Geometry: final body of the model. Coordinates: model frame, mm. A direction names the side the tool comes from. Give positions to 0.01 mm unless a question says otherwise; leave off trailing zeros. Write each loop counter-clockwise with the first axis right and the second up, starting at its lowest first coordinate (ties: lowest second). Pieces come first, ordered by that corner, then holes. Notation, with made-up numbers: M 1.25,5 L 22.25,5 A8 cw 22.25,14 Z; hole C 52,19 d1. An arc over 180 degrees is marked long. Answer as a JSON object with one key per item and string values.
Autodesk Inventor part; units mm, degrees
ref_plane "YZ Plane" through (0, 0, 0) normal (1, 0, 0) x (0, 1, 0)
ref_plane "XZ Plane" through (0, 0, 0) normal (0, 1, 0) x (-1, 0, 0)
ref_plane "XY Plane" through (0, 0, 0) normal (0, 0, 1) x (1, 0, 0)
sketch "スケッチ1" plane through (0, 0, 0) normal (0, 1, 0) x (-1, 0, 0)
  line L0 (-88.25, 46.25) -> (88.25, 46.25)
  line L1 (88.25, 46.25) -> (88.25, -46.25)
  line L2 (88.25, -46.25) -> (-88.25, -46.25)
  line L3 (-88.25, -46.25) -> (-88.25, 46.25)
  line L4 (-88.25, 46.25) -> (88.25, -46.25) construction
  line L5 (88.25, 46.25) -> (-88.25, -46.25) construction
  circle A0 centre (84.75, 42.75) radius 1.55
  circle A1 centre (9.75, 42.75) radius 1.55
  circle A2 centre (-84.75, 42.75) radius 1.55
  line L6 (151.0272, 0) -> (-157.6431, 0) construction
  line L7 (0, 129.3763) -> (0, -94.6315) construction
  circle A3 centre (84.75, -42.75) radius 1.55
  circle A4 centre (9.75, -42.75) radius 1.55
  circle A5 centre (-84.75, -42.75) radius 1.55
  circle A6 centre (30, -25.75) radius 1.55
  circle A7 centre (30, -16.25) radius 1.55
  line L8 (88.25, -25.75) -> (-88.25, -25.75) construction
  line L9 (-88.25, -16.25) -> (88.25, -16.25) construction
  circle A8 centre (-69.5, -25.75) radius 1.55
  circle A9 centre (-69.5, -16.25) radius 1.55
  circle A10 centre (84.75, -29.75) radius 1.55
  circle A11 centre (84.75, -14.75) radius 1.55
  circle A12 centre (84.75, 0.25) radius 1.55
  circle A13 centre (84.75, 15.25) radius 1.55
  circle A14 centre (84.75, 30.25) radius 1.55
  circle A15 centre (76.5, -25.75) radius 1.55
  circle A16 centre (76.5, -13.75) radius 1.55
  circle A17 centre (76.5, -1.75) radius 1.55
  circle A18 centre (76.5, 10.25) radius 1.55
  line L10 (-55.5, -30.75) -> (24.5, -30.75)
  line L11 (24.5, -30.75) -> (24.5, 29.25)
  line L12 (24.5, 29.25) -> (-55.5, 29.25)
  line L13 (-55.5, 29.25) -> (-55.5, -30.75)
  line L14 (-55.5, -30.75) -> (24.5, 29.25) construction
  line L15 (24.5, -30.75) -> (-55.5, 29.25) construction
  point P0 (0, 0)
  point P1 (-15.5, -0.75)
  dimension "d105" = 176.5
  dimension "d106" = 92.5
  dimension "d107" = 3.5
  dimension "d108" = 3.5
  dimension "d109" = 3.1
  dimension "d110" = 78.5
  dimension "d111" = 3.5
  dimension "d112" = 3.1
  dimension "d113" = 173
  dimension "d114" = 3.5
  dimension "d115" = 3.1
  dimension "d116" = 46.25
  dimension "d117" = 88.25
  dimension "d118" = 58.25
  dimension "d119" = 20.5
  dimension "d120" = 30
  dimension "d121" = 3.1
  dimension "d122" = 3.1
  dimension "d123" = 58.25
  dimension "d129" = 3.1
  dimension "d130" = 3.1
  dimension "d132" = 9.5
  dimension "d133" = 20.5
  dimension "d134" = 30
  dimension "d136" = 16.5
  dimension "d137" = 3.5
  dimension "d138" = 3.1
  dimension "d141" = 15
  dimension "d146" = 20.5
  dimension "d147" = 11.75
  dimension "d148" = 3.1
  dimension "d151" = 12
  dimension "d156" = 15.5
  dimension "d157" = 75.5
  dimension "d158" = 63.75
  dimension "d159" = 143.75
  dimension "d164" = 99.5
  dimension "d165" = 157.75
extrude "押し出し1" add sketch "スケッチ1" along normal blind 3
fillet "フィレット1" radius 2 4 edges at (-24.5, 1.5, 29.25) (-24.5, 1.5, -30.75) (55.5, 1.5, 29.25) (55.5, 1.5, -30.75)
fillet "フィレット2" radius 3 4 edges at (-88.25, 1.5, 46.25) (-88.25, 1.5, -46.25) (88.25, 1.5, 46.25) (88.25, 1.5, -46.25)
equation "\"d108\" = d107"
equation "\"d111\" = d107"
equation "\"d112\" = d109"
equation "\"d114\" = d111"
equation "\"d115\" = d112"
equation "\"d121\" = d109"
equation "\"d122\" = d109"
equation "\"d123\" = d118"
equation "\"d129\" = d131"
equation "\"d130\" = d131"
equation "\"d138\" = d109"
equation "\"d148\" = d138"
properties part number "Sole" material "GFRC"
1) Line query: line 1 (Z direction, x = 69.5, y = 2.1); line 2 (Z direction, x = -76.5, y = 2.2); line 3 (X direction, y = 0.2, z = 30). Output: solid intervals per line, ascending. Write a range as from..to.
Geometry check:
{"line 1": "z = -46.25..-27.3, -24.2..-17.8, -14.7..46.25", "line 2": "z = -46.25..-27.3, -24.2..-15.3, -12.2..-3.3, -0.2..8.7, 11.8..46.25", "line 3": "x = -88.25..-86.28, -83.22..88.25"}
2) Cut plane A-A on z = 19. Return loops of the section in (x, y), and give its area (4 significant figures).
Geometry check:
{"outline": "M -88.25,0 L -24.5,0 L -24.5,3 L -88.25,3 Z; M 55.5,0 L 88.25,0 L 88.25,3 L 55.5,3 Z", "area": "289.5 mm2"}
3) Cut plane B-B on x = 0.5. Return loops of the section in (y, z).
Geometry check:
{"outline": "M 0,-46.25 L 3,-46.25 L 3,-30.75 L 0,-30.75 Z; M 0,29.25 L 3,29.25 L 3,46.25 L 0,46.25 Z"}
4) Contact query for a flat-ended pin moving along its axis: P1, Ø3, axis at x = 69.5, z = -16.25, coming from the -Y side. Output: stop coordinate, or through.
Geometry check:
{"P1": "passes through"}
5) Cut plane C-C on y = 2.05. Give the number of separate pieces and of enclosed holes in the cut face, and give its area (3 significant figures).
Geometry check:
{"separate pieces": "1", "enclosed holes": "20", "area": "11,400 mm2"}
6) Set-up query: faces 1 (the flat face through (-24.5, 1, -1)), 2 (the flat face through (-88.25, 1, 1)). Return all of +Z, -Z, +X, -X, +Y, -Y with unobstructed straight access to the full face (end or side cutting, diameter ignored); none if empty.
Geometry check:
{"face 1": "+Y, -Y", "face 2": "+Z, -Z, -X, +Y, -Y"}
7) Pull-direction query (X, two-part tool) for faces 3 (the cylindrical face through (87.35, 1.52, 45.39)), 4 (the cylindrical face through (84.035, 1.479, -41.375)), 5 (the cylindrical face through (-87.39, 1.52, 45.35)); classes: pulls with the +X half, pulls with the -X half, needs draft (parallel to the pull), parting line crosses it, or undercut.
Geometry check:
{"face 3": "pulls with the +X half", "face 4": "undercut", "face 5": "pulls with the -X half"}
